Could you check a few things on this drawing? It's one solid part, dimensions in mm from its lowest x, y, z. A direction names the side the tool comes from. Round coordinates to 2 decimals unless told otherwise and drop trailing zeros. Write each loop counter-clockwise with the first axis right and the second up, starting at its lowest first coordinate (ties: lowest second). Pieces come first, ordered by that corner, then holes. Notation, with made-up numbers: (73, 60.25) -> (99, 60.25) arc R27 ccw to (99, 86.25) -> close; hole circle Ø11 at (-37.5, -16). An arc over 180 degrees is marked (long way). Answer as CSV lines item,"result".
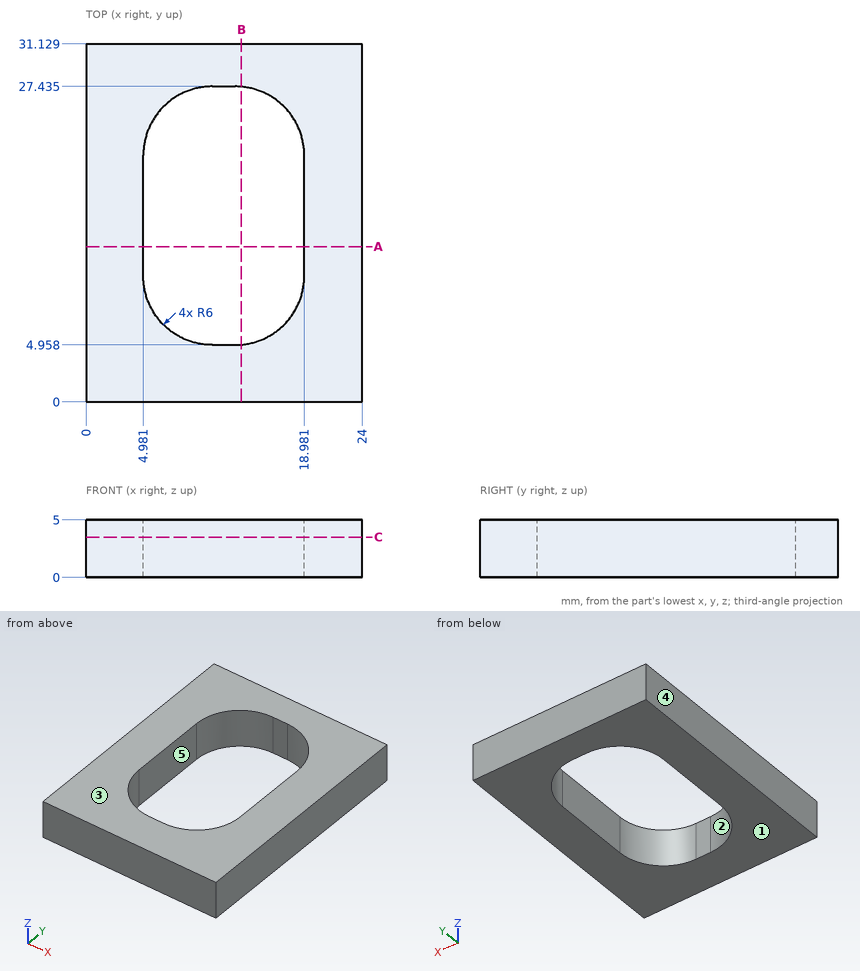
1. Suppose I cut it at A-A on y = 13.5. Please give me the cut outline in (x, z), and give its area (3 significant figures).
Numbers:
outline,"(0, 0) -> (4.98, 0) -> (4.98, 5) -> (0, 5) -> close; (18.98, 0) -> (24, 0) -> (24, 5) -> (18.98, 5) -> close"
area,"50.0 mm^2"
2. Suppose I cut it at B-B on x = 13.5. Please give me the cut outline in (y, z).
Numbers:
outline,"(0, 0) -> (4.98, 0) -> (4.98, 5) -> (0, 5) -> close; (27.41, 0) -> (31.13, 0) -> (31.13, 5) -> (27.41, 5) -> close"
3. On a 3-axis mill with a long thin cutter (end or side, diameter ignored), from which of +Z, -Z, +X, -X, +Y, -Y can I reach the whole of each face in a straight line? I mean the marked faces 1 and 2. Say none if no direction works.
Numbers:
face 1,"-Z, +X, -X, +Y, -Y"
face 2,"+Z, -Z"
4. Suppose I cut it at C-C on z = 3.5. Please give me the cut outline in (x, y) (1 decimal).
Numbers:
outline,"(0, 0) -> (24, 0) -> (24, 31.1) -> (0, 31.1) -> close; hole (5, 11) arc R6 ccw to (11, 5) -> (13, 5) arc R6 ccw to (19, 11) -> (19, 21.4) arc R6 ccw to (13, 27.4) -> (11, 27.4) arc R6 ccw to (5, 21.4) -> close"
5. If I drill on line 1 (X direction, y = 17.5, z = 3.95); line 2 (Y direction, x = 11.5, z = 2.7) (1 decimal); line 3 (Y direction, x = 15.25, z = 2.85), over which ranges is the centre line in solid material (lowest first)?
Numbers:
line 1,"x = 0 to 4.98, 18.98 to 24"
line 2,"y = 0 to 5, 27.4 to 31.1"
line 3,"y = 0 to 5.4, 26.99 to 31.13"
6. If we mould it in two halves opening along X, with no side actions, what happens to the marked faces 3, 4 and 5? For each: released by +X, released by -X, zero draft, split by the parting line, or undercut.
Numbers:
face 3,"zero draft"
face 4,"released by -X"
face 5,"undercut"
